from build123d import *

# Parameters (mm, degrees)
BOSS_EXTRU_1_DEPTH      = 169
ESQUISSE2_R             = 3.307300662
ENL_V_MAT_EXTRU_1_DEPTH = 22
ESQUISSE3_R             = 3
BOSS_EXTRU_3_DEPTH      = 12
ESQUISSE4_R             = 3
BOSS_EXTRU_4_DEPTH      = 12
ESQUISSE5_R             = 3
ENL_V_MAT_EXTRU_2_DEPTH = 22


with BuildPart() as part:
    # Esquisse1 → Boss.-Extru.1 (new body)
    with BuildSketch(Plane.XY):
        with BuildLine():
            Line((0, 0), (60, 0))
            Line((60, 0), (60, -35))
            ThreePointArc((60, -35), (25.240598959, -25.658973212), (0, 0))
        make_face()
    extrude(amount=BOSS_EXTRU_1_DEPTH)

    # Esquisse2 → Enlèv. mat.-Extru.1 (cut)
    with BuildSketch(Plane(origin=(0, 0, 0), x_dir=(-1, 0, 0), z_dir=(0, 0, -1))):
        with Locations((-31, -12)):
            Circle(ESQUISSE2_R)
    extrude(amount=-ENL_V_MAT_EXTRU_1_DEPTH, mode=Mode.SUBTRACT)

    # Esquisse3 → Boss.-Extru.3 (add)
    with BuildSketch(Plane(origin=(0, 0, 0), x_dir=(1, 0, 0), z_dir=(0, 1, 0))):
        with Locations(Location((38, -42.5, 0), (0, 0, 90))):
            Circle(ESQUISSE3_R)
    extrude(amount=BOSS_EXTRU_3_DEPTH)

    # Esquisse4 → Boss.-Extru.4 (add)
    with BuildSketch(Plane(origin=(0, 0, 0), x_dir=(1, 0, 0), z_dir=(0, 1, 0))):
        with Locations(Location((38, -126.5, 0), (0, 0, 90))):
            Circle(ESQUISSE4_R)
    extrude(amount=BOSS_EXTRU_4_DEPTH)

    # Esquisse5 → Enlèv. mat.-Extru.2 (cut)
    with BuildSketch(Plane.XY.offset(169)):
        with Locations((31, -11.770310322)):
            Circle(ESQUISSE5_R)
    extrude(amount=-ENL_V_MAT_EXTRU_2_DEPTH, mode=Mode.SUBTRACT)


solid = part.part
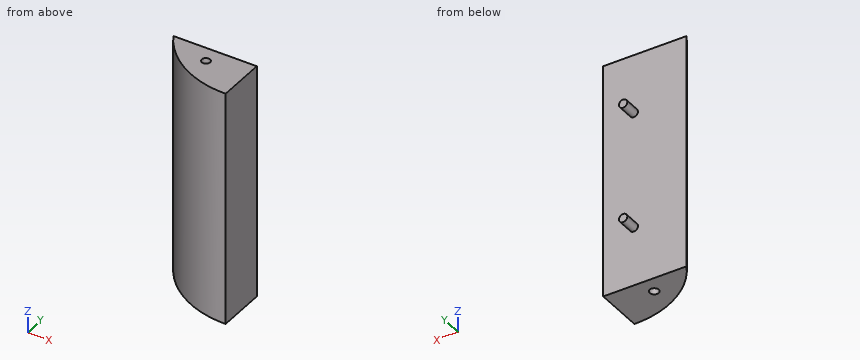
CAD build for the part. Positions are in the model's coordinates, mm. Coordinates: 2 decimals unless noted, no trailing zeros. Order: outer loops, then holes, each group sorted by start corner. A loop starts at its lowest first (then second) coordinate and runs counter-clockwise, first axis right, second up.
Item 1: Band-saw the part on C-C on z = 126.5. List the corners of the cut face in (x, y).
Check sheet entries:
outline: (0, 0) arc R68.57 ccw to (60, -35) - (60, 0) - (41, 0) - (41, 12) - (35, 12) - (35, 0) - close
Item 2: Band-saw the part on D-D on x = 31. List the corners of the cut face in (y, z), plus the area to 3 significant figures.
Check sheet entries:
outline: (-28.66, 0) - (-15.31, 0) - (-15.31, 22) - (-8.69, 22) - (-8.69, 0) - (0, 0) - (0, 169) - (-8.77, 169) - (-8.77, 147) - (-14.77, 147) - (-14.77, 169) - (-28.66, 169) - close
area: 4,570 mm2
Item 3: Band-saw the part on A-A on y = 6. List the corners of the cut face in (x, z).
Check sheet entries:
outline: circle Ø6 at (38, 42.5); circle Ø6 at (38, 126.5)
Item 4: Pin check, flat tips, straight feed: pin 1 Ø3 at (x, z) = (26, 29.5) entering from -Y; pin 2 Ø3 at (x, z) = (9.5, 55.5) entering from -Y; pin 3 Ø1 at (x, z) = (12.5, 124.5) entering from -Y. Stop position of each tip, or through.
Check sheet entries:
pin 1: stops at y = -26.92
pin 2: stops at y = -14.61
pin 3: stops at y = -16.55
Item 5: Drill centre lines: L1, parallel to Y at x = 31, z = 16.25; L2, parallel to X at y = -1, z = 97; L3, parallel to Y at x = 12.5, z = 78. Where is each one in solid material? Low to high.
Check sheet entries:
L1: y = -28.66 to -15.31, -8.69 to 0
L2: x = 0.57 to 60
L3: y = -16.08 to 0
Item 6: Band-saw the part on B-B on z = 17. List the corners of the cut face in (x, y), plus the area to 3 significant figures.
Check sheet entries:
outline: (0, 0) arc R68.57 ccw to (60, -35) - (60, 0) - close; hole circle Ø6.61 at (31, -12)
area: 1,460 mm2
